```python
from build123d import *

# Parameters (mm, degrees)
F2_R = 5


with BuildPart() as f1:
    # F0 (on Front) → F1 (revolve)
    with BuildSketch(Plane.XZ):
        Polygon((-22.704557, -50), (-22, -50), (-18, -15), (-19, -8), (-15, -4), (-15, 0), (-15.7, 0), (-15.7, -3.710051), (-19.742462, -7.752513), (-18.70569, -15.009917), align=None)
        Polygon((-15.7, 0), (-15, 0), (-15, 4), (-19, 8), (-18, 15), (-22, 50), (-22.704557, 50), (-18.70569, 15.009917), (-19.742462, 7.752513), (-15.7, 3.710051), align=None)
    revolve(axis=Axis((0, 0, -25), (0, 0, -1)))

    # F2
    f2_edges = [f1.edges().sort_by_distance(p)[0] for p in [
        (19.742462, 0, 7.752513),
        (19, 0, 8),
        (18, 0, 15),
        (18.70569, 0, 15.009917),
        (15.7, 0, -3.710051),
        (19.742462, 0, -7.752513),
        (18.70569, 0, -15.009917),
        (18, 0, -15),
        (19, 0, -8),
        (15, 0, -4),
        (15.7, 0, 3.710051),
        (-15, 0, 0),
        (15, 0, 4),
    ]]
    fillet(f2_edges, radius=F2_R)


solid = f1.part
```
The listing builds one solid part. Answer for the finished solid, in the listing's coordinates (mm). A direction names the side the tool comes from. Give positions to 0.01 mm unless a question says otherwise; leave off trailing zeros. Order: outer loops, then holes, each group sorted by start corner. A loop starts at its lowest first (then second) coordinate and runs counter-clockwise, first axis right, second up.
1) Find section A-A on z = 28. Write down the section's boundary in (x, y), then the cut area to 3 significant figures.
Reported:
outline: circle Ø40.38 at (0, 0); hole circle Ø38.97 at (0, 0)
area: 87.8 mm2
2) For faces 1 (the face through (-8, -15, -6)), 2 (the face through (4.4, -19.8, 28.8)), determine the directions among +Z, -Z, +X, -X, +Y, -Y from which every point of the face is accessible in a straight line to the end or side of a thin tool.
Reported:
face 1: -Z
face 2: none
3) Find section B-B on z = 39. Write down the section's boundary in (x, y), then the cut area to 3 significant figures.
Reported:
outline: circle Ø42.89 at (0, 0); hole circle Ø41.49 at (0, 0)
area: 93.4 mm2
4) Determine the mould class of faces 3 (the face through (12, 19, -50)), 4 (the face through (2.044, 15.566, -0.023)), 5 (the face through (-8.36, -16.074, 14.175)) for opening direction Y: pulls with the +Y half, pulls with the -Y half, needs draft (parallel to the pull), parting line crosses it, or undercut.
Reported:
face 3: needs draft
face 4: parting line crosses it
face 5: undercut
5) Given P1, Ø3, axis at x = -15, z = -5, coming from the -Y side; P2, Ø3, axis at x = -13, z = -31, coming from the +Y side; P3, Ø1, axis at y = -6.5, z = 20.5, coming from the +X side, each flat-ended and moving along its own axis, determine where each tip first touches the part or whether it passes through.
Reported:
P1: stops at y = -11.48
P2: stops at y = 17.03
P3: stops at x = 18.39
6) Consider line 1 along X through (y, z) = (0, -0.4); line 2 along Y through (x, z) = (-7.5, 35). Determine where each line is inside the solid, lowest interval first.
Reported:
line 1: x = -15.7 to -15, 15 to 15.7
line 2: y = -19.6 to -18.85, 18.85 to 19.6
